Drawing for the job (mm, zero at the part's lowest x, y, z). Round coordinates to 2 decimals unless told otherwise and drop trailing zeros. Loops run counter-clockwise (first coordinate to the right, second up) from the corner with the lowest first, then second, coordinate; pieces in that order, holes last. Notation, with made-up numbers: M 73,17 L 122,17 A25 cw 122,48 Z; hole C 0.25,-38 d6. An arc over 180 degrees is marked long. Answer in a Markdown table with one row per item.
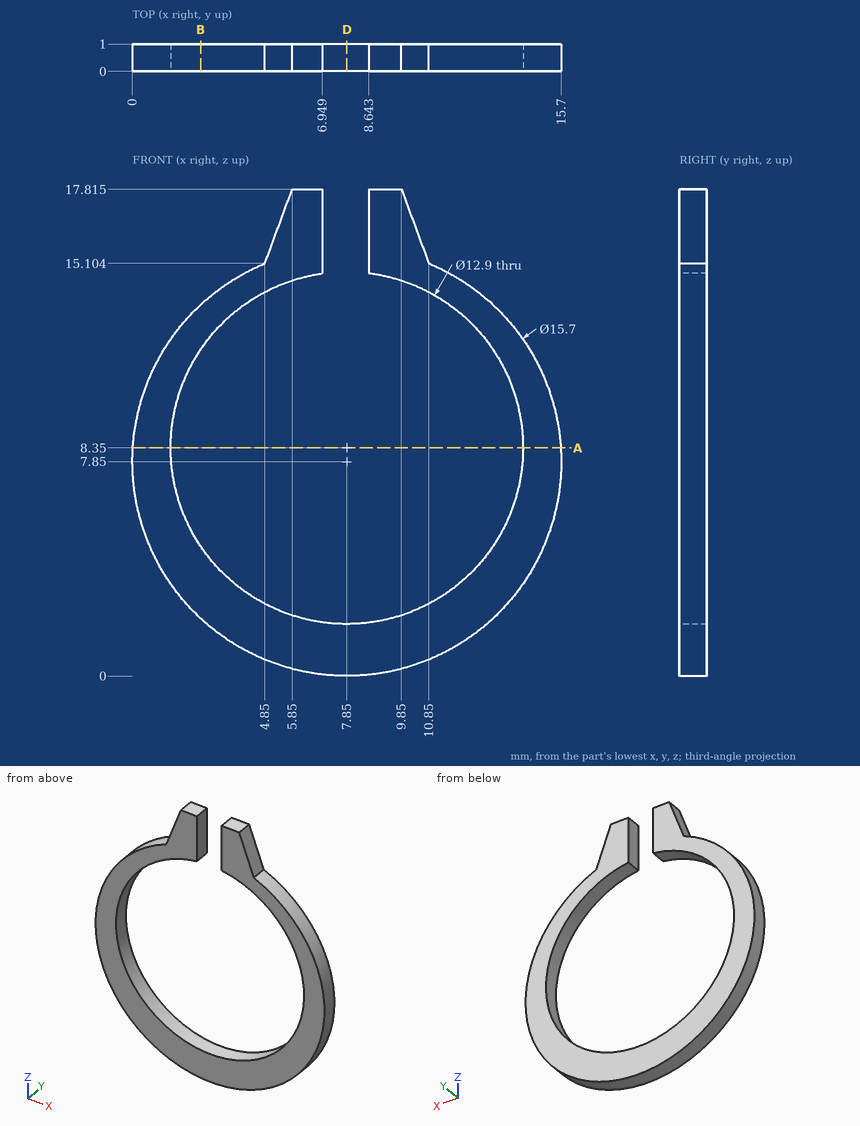
1. Wall check: probe 1 along Z at (x, y) = (8, 0.1); probe 2 along X at (y, z) = (0.8, 8.35); probe 3 along X at (y, z) = (0.55, 9.5) (1 decimal). Give the ranges that are in metal, low to high.
Verdict:
| item | result |
|---|---|
| probe 1 | z = 0 to 1.9 |
| probe 2 | x = 0.02 to 1.4, 14.3 to 15.68 |
| probe 3 | x = 0.2 to 1.5, 14.2 to 15.5 |
2. Saw through at A-A (z = 8.35). Write the cut outline in (x, y).
Verdict:
| item | result |
|---|---|
| outline | M 0.02,0 L 1.4,0 L 1.4,1 L 0.02,1 Z; M 14.3,0 L 15.68,0 L 15.68,1 L 14.3,1 Z |
3. Pin check, flat tip, straight feed: pin 1 (4 mm diameter, centred on x = 7.5, z = 13, fed in from +Y). Stop position of the tip, or through.
Verdict:
| item | result |
|---|---|
| pin 1 | stops at y = 1 |
4. Saw through at B-B (x = 2.5). Write the cut outline in (y, z) (1 decimal).
Verdict:
| item | result |
|---|---|
| outline | M 0,2.1 L 1,2.1 L 1,4.7 L 0,4.7 Z; M 0,12 L 1,12 L 1,13.6 L 0,13.6 Z |
5. Saw through at D-D (x = 7.85). Write the cut outline in (y, z).
Verdict:
| item | result |
|---|---|
| outline | M 0,0 L 1,0 L 1,1.9 L 0,1.9 Z |
